from build123d import *

# Parameters (mm, degrees)
SKETCH1_W                 = 48.641
SKETCH1_H                 = 14.859
BOSS_EXTRUDE1_DEPTH       = 9.398
SKETCH2_W                 = 6.35
SKETCH2_H                 = 13.335
CUT_EXTRUDE1_DEPTH        = 51.65421707
F_5_CLEARANCE_HOLE1_D     = 3.556
F_5_CLEARANCE_HOLE1_DEPTH = 1.524
F_5_CLEARANCE_HOLE2_D     = 3.556
F_5_CLEARANCE_HOLE2_DEPTH = 14.859
F_5_CLEARANCE_HOLE3_D     = 3.556
FILLET1_R                 = 0.635


with BuildPart() as part:
    # Sketch1 → Boss-Extrude1 (new body)
    with BuildSketch(Plane(origin=(-4.699, 0, 0), x_dir=(0, -1, 0), z_dir=(-1, 0, 0))):
        with Locations((-24.3205, -5.9055)):
            Rectangle(SKETCH1_W, SKETCH1_H)
    extrude(amount=-BOSS_EXTRUDE1_DEPTH)

    # Sketch2 → Cut-Extrude1 (cut, through all)
    with BuildSketch(Plane.XZ):
        with Locations((0, -6.6675)):
            Rectangle(SKETCH2_W, SKETCH2_H)
    extrude(amount=-CUT_EXTRUDE1_DEPTH, mode=Mode.SUBTRACT)

    # #5 Clearance Hole1
    with Locations(Plane(origin=(4.699, 0, 0), x_dir=(0, 0, -1), z_dir=(1, 0, 0))):
        with Locations((8.5725, 34.0995), (8.5725, 43.8785), (8.5725, 24.3205), (8.5725, 14.5415), (8.5725, 4.7625)):
            Hole(F_5_CLEARANCE_HOLE1_D / 2, depth=F_5_CLEARANCE_HOLE1_DEPTH)

    # #5 Clearance Hole2
    with Locations(Plane.XY.offset(1.524)):
        with Locations((0, 34.0995), (0, 43.8785), (0, 24.3205), (0, 14.5415), (0, 4.7625)):
            Hole(F_5_CLEARANCE_HOLE2_D / 2, depth=F_5_CLEARANCE_HOLE2_DEPTH)

    # #5 Clearance Hole3 (through all)
    with Locations(Plane(origin=(-3.175, 0, 0), x_dir=(0, 0, -1), z_dir=(1, 0, 0))):
        with Locations((8.5725, 34.0995), (8.5725, 43.8785), (8.5725, 24.3205), (8.5725, 14.5415), (8.5725, 4.7625)):
            Hole(F_5_CLEARANCE_HOLE3_D / 2)

    # Fillet1
    fillet1_edges = [part.edges().sort_by_distance(p)[0] for p in [
        (-3.937, 48.641, -13.335),
        (-3.937, 0, -13.335),
        (3.937, 0, -13.335),
        (3.937, 48.641, -13.335),
    ]]
    fillet(fillet1_edges, radius=FILLET1_R)


solid = part.part
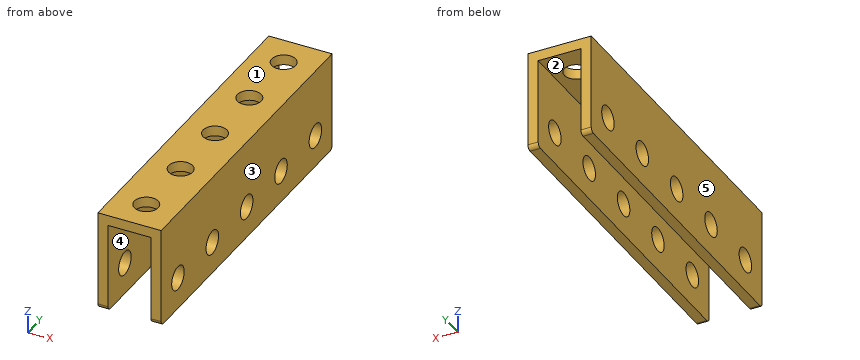
The model under review builds one solid part; all positions refer to its coordinate system, in mm. Face numbers are marked on the shaded views. A direction names the side the tool comes from. Coordinates: 2 decimals unless noted, no trailing zeros. Loops run counter-clockwise (first coordinate to the right, second up) from the corner with the lowest first, then second, coordinate; pieces in that order, holes last. Notation, with made-up numbers: (28.25, 37) -> (55.25, 37) arc R29 cw to (55.25, 72) -> close; hole circle Ø5 at (-17, 49). An arc over 180 degrees is marked (long way). Use a Markdown table: item, result. Add a question column.
1. Add section B-B on z = -1. Write out the cut boundary in (x, y) (3 decimals).
2. To check wall thickness, follow line 1 (Y direction, x = 0, z = 0.7); line 2 (X direction, y = 30, z = -11) (3 decimals); line 3 (Y direction, x = 3.75, z = -7.5). State the ranges of each line that lie inside material, in increasing order.
3. Add section A-A on x = 0. Write out the cut boundary in (y, z).
4. Add section D-D on y = 29. Write out the cut boundary in (x, z) (3 decimals), plus the area to 3 significant figures.
5. Add section C-C on y = 44.5. Write out the cut boundary in (x, z) (3 decimals).
6. Draft analysis for pull direction X (two halves, no side actions). For the marked faces 3, 4 and 5, state which applies: pulls with the +X half, pulls with the -X half, needs draft (parallel to the pull), parting line crosses it, or undercut.
7. Clearance check with a flat-ended pin moving along its axis: pin 1 Ø1.9 at (x, y) = (1, 36.5) entering from -Z. State where the tip first meets the part, or that it passes through.
8. Machinability: for the marked faces 1 and 2, which of the approach directions +Z, -Z, +X, -X, +Y, -Y give a long, thin tool a straight path to every point of the face, cutting with its end or side? Answer none if there is none.
Returned:
| question | item | result |
|---|---|---|
| 1 | outline | (-4.699, 0) -> (-3.175, 0) -> (-3.175, 48.641) -> (-4.699, 48.641) -> close; (3.175, 0) -> (4.699, 0) -> (4.699, 48.641) -> (3.175, 48.641) -> close |
| 2 | line 1 | y = 0 to 2.98, 6.54 to 12.76, 16.32 to 22.54, 26.1 to 32.32, 35.88 to 42.1, 45.66 to 48.64 |
| 2 | line 2 | x = -4.699 to -3.175, 3.175 to 4.699 |
| 2 | line 3 | y = 0 to 3.34, 6.18 to 13.12, 15.96 to 22.9, 25.74 to 32.68, 35.52 to 42.46, 45.3 to 48.64 |
| 3 | outline | (0, 0) -> (2.98, 0) -> (2.98, 1.52) -> (0, 1.52) -> close; (6.54, 0) -> (12.76, 0) -> (12.76, 1.52) -> (6.54, 1.52) -> close; (16.32, 0) -> (22.54, 0) -> (22.54, 1.52) -> (16.32, 1.52) -> close; (26.1, 0) -> (32.32, 0) -> (32.32, 1.52) -> (26.1, 1.52) -> close; (35.88, 0) -> (42.1, 0) -> (42.1, 1.52) -> (35.88, 1.52) -> close; (45.66, 0) -> (48.64, 0) -> (48.64, 1.52) -> (45.66, 1.52) -> close |
| 4 | outline | (-4.699, -13.335) -> (-3.175, -13.335) -> (-3.175, 0) -> (3.175, 0) -> (3.175, -13.335) -> (4.699, -13.335) -> (4.699, 1.524) -> (-4.699, 1.524) -> close |
| 4 | area | 55.0 mm² |
| 5 | outline | (-4.699, -13.335) -> (-3.175, -13.335) -> (-3.175, -10.238) -> (-4.699, -10.238) -> close; (-4.699, -6.907) -> (-3.175, -6.907) -> (-3.175, 0) -> (-1.666, 0) -> (-1.666, 1.524) -> (-4.699, 1.524) -> close; (1.666, 0) -> (3.175, 0) -> (3.175, -6.907) -> (4.699, -6.907) -> (4.699, 1.524) -> (1.666, 1.524) -> close; (3.175, -13.335) -> (4.699, -13.335) -> (4.699, -10.238) -> (3.175, -10.238) -> close |
| 6 | face 3 | pulls with the +X half |
| 6 | face 4 | undercut |
| 6 | face 5 | pulls with the -X half |
| 7 | pin 1 | stops at z = 0 |
| 8 | face 1 | +Z, +X, -X, +Y, -Y |
| 8 | face 2 | -Z, +Y, -Y |
